Check sheet for the modelled part. Datum: model origin and axes. Units: mm. Round coordinates to 2 decimals unless told otherwise and drop trailing zeros. Order: outer loops, then holes, each group sorted by start corner. A loop starts at its lowest first (then second) coordinate and runs counter-clockwise, first axis right, second up.
(1) Sectioned sample at C-C, the plane y = -8.5. Enter the section's corners in (x, z), and give its area (3 significant figures).
(2) Thickness scan on probe 1 along Y at (x, z) = (0, 1); probe 2 along Y at (x, z) = (6.25, 0.3); probe 3 along Y at (x, z) = (-7.5, 2.15). Record the ranges inside material, lowest first.
(3) Sectioned sample at A-A, the plane y = -1. Enter the section's corners in (x, z), and give its area (3 significant figures).
(4) Sectioned sample at B-B, the plane z = 2.15. Count the separate pieces of the cut face and the enclosed holes in it, and give its area (3 significant figures).
(5) Depth check by flat-ended pin: pin 1 (1.4 mm diameter, centred on x = 7.5, y = -8.5, fed in from -Z) (1 decimal); pin 2 (1.5 mm diameter, centred on y = 28.5, z = 2, fed in from -X); pin 3 (1.5 mm diameter, centred on x = -2.5, y = -9.5, fed in from -Z); pin 4 (0.9 mm diameter, centred on x = 13, z = 2, fed in from -Y). Enter the tip coordinate at first touch or a pass-through.
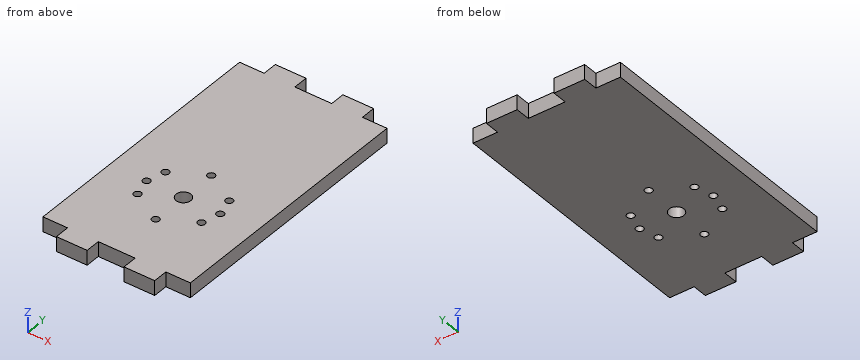
```python
from build123d import *

# Parameters (mm, degrees)
SKETCH1_R           = 0.75
SKETCH1_R_2         = 1.5
BOSS_EXTRUDE1_DEPTH = 3


with BuildPart() as part:
    # Sketch1 → Boss-Extrude1 (new body)
    with BuildSketch(Plane.XY):
        Polygon((-15, 26.5), (-10, 26.5), (-10, 29.5), (-3.75, 29.5), (-3.75, 26.5), (3.75, 26.5), (3.75, 29.5), (10, 29.5), (10, 26.5), (15, 26.5), (15, -26.5), (10, -26.5), (10, -29.5), (3.75, -29.5), (3.75, -26.5), (-3.75, -26.5), (-3.75, -29.5), (-10, -29.5), (-10, -26.5), (-15, -26.5), align=None)
        with Locations((0, -1)):
            Circle(SKETCH1_R, mode=Mode.SUBTRACT)
        with Locations((6.495190528, -4.75)):
            Circle(SKETCH1_R, mode=Mode.SUBTRACT)
        with Locations((6.495190528, -12.25)):
            Circle(SKETCH1_R, mode=Mode.SUBTRACT)
        with Locations((0, -16)):
            Circle(SKETCH1_R, mode=Mode.SUBTRACT)
        with Locations((-6.495190528, -12.25)):
            Circle(SKETCH1_R, mode=Mode.SUBTRACT)
        with Locations((-6.495190528, -4.75)):
            Circle(SKETCH1_R, mode=Mode.SUBTRACT)
        with Locations((0, -8.5)):
            Circle(SKETCH1_R_2, mode=Mode.SUBTRACT)
        with Locations((-7.5, -8.5)):
            Circle(SKETCH1_R, mode=Mode.SUBTRACT)
        with Locations((7.5, -8.5)):
            Circle(SKETCH1_R, mode=Mode.SUBTRACT)
    extrude(amount=BOSS_EXTRUDE1_DEPTH)


solid = part.part
```
Derived:
1. outline: (-15, 0) - (-8.25, 0) - (-8.25, 3) - (-15, 3) - close; (-6.75, 0) - (-1.5, 0) - (-1.5, 3) - (-6.75, 3) - close; (1.5, 0) - (6.75, 0) - (6.75, 3) - (1.5, 3) - close; (8.25, 0) - (15, 0) - (15, 3) - (8.25, 3) - close
1. area: 72.0 mm2
2. probe 1: y = -26.5 to -16.75, -15.25 to -10, -7 to -1.75, -0.25 to 26.5
2. probe 2: y = -29.5 to -12.96, -11.54 to -5.46, -4.04 to 29.5
2. probe 3: y = -29.5 to -9.25, -7.75 to 29.5
3. outline: (-15, 0) - (-0.75, 0) - (-0.75, 3) - (-15, 3) - close; (0.75, 0) - (15, 0) - (15, 3) - (0.75, 3) - close
3. area: 85.5 mm2
4. separate pieces: 1
4. enclosed holes: 9
4. area: 1,640 mm2
5. pin 1: passes through
5. pin 2: stops at x = -10
5. pin 3: stops at z = 0
5. pin 4: stops at y = -26.5
